```python
from build123d import *

# Parameters (mm, degrees)
F0_W      = 381
F0_H      = 609.6
F1_DEPTH  = 127
F2_T      = -1.5748
F3_W      = 1.5748
F3_H      = 606.4504
F4_DEPTH  = 125.4252
F5_W      = 63.5
F5_H      = 63.5
F6_DEPTH  = 127
F7_W      = 63.5
F7_H      = 63.5
F8_DEPTH  = 128.5748
F9_R      = 22.479
F10_DEPTH = 41.148
F11_R     = 15.875
F12_DEPTH = 42.7228


with BuildPart() as f1:
    # F0 (on Top) → F1 (new body)
    with BuildSketch(Plane.XY):
        with Locations((190.5, 304.8)):
            Rectangle(F0_W, F0_H)
    extrude(amount=F1_DEPTH)

    # F2
    f2_openings = [f1.faces().sort_by_distance(p)[0] for p in [
        (190.5, 304.8, 127),
    ]]
    offset(amount=F2_T, openings=f2_openings)

    # F3 (on face) → F4 (join, through all)
    with BuildSketch(Plane.XY.offset(1.5748)):
        with Locations((129.3622, 304.8)):
            Rectangle(F3_W, F3_H)
        with Locations((256.3622, 304.8)):
            Rectangle(F3_W, F3_H)
    extrude(amount=F4_DEPTH)

    # F5 (on face) → F6 (cut, through all)
    with BuildSketch(Plane.YZ.offset(257.1496)):
        with Locations((33.3248, 33.3248)):
            Rectangle(F5_W, F5_H)
    extrude(amount=-F6_DEPTH, mode=Mode.SUBTRACT)

    # F7 (on face) → F8 (cut, through all)
    with BuildSketch(Plane.YZ.offset(130.1496)):
        with Locations((576.2752, 33.3248)):
            Rectangle(F7_W, F7_H)
    extrude(amount=-F8_DEPTH, mode=Mode.SUBTRACT)

    # F9 (on face) → F10 (join)
    with BuildSketch(Plane(origin=(0, 0, 0), x_dir=(0, -1, 0), z_dir=(-1, 0, 0))):
        with Locations((-22.479, 22.479)):
            Circle(F9_R)
    extrude(amount=F10_DEPTH)

    # F11 (on face) → F12 (cut, through all)
    with BuildSketch(Plane(origin=(-41.148, 0, 0), x_dir=(0, -1, 0), z_dir=(-1, 0, 0))):
        with Locations((-22.479, 22.479)):
            Circle(F11_R)
    extrude(amount=-F12_DEPTH, mode=Mode.SUBTRACT)


solid = f1.part
```
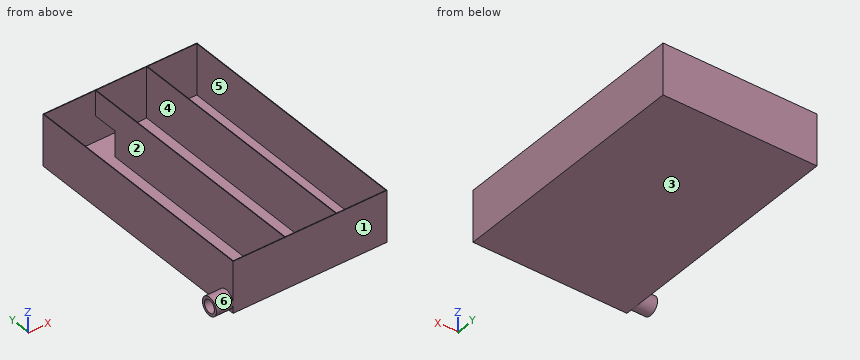
Here's how the part is built. I have some questions about the finished solid (model axes, mm). Face numbers are marked on the shaded views. A direction names the side the tool comes from. Give positions to 0.01 mm unless a question says otherwise; leave off trailing zeros. Write each loop counter-clockwise with the first axis right and the second up, starting at its lowest first coordinate (ties: lowest second). Pieces come first, ordered by that corner, then holes. Notation, with made-up numbers: (88, 40.5) -> (134, 40.5) arc R29 cw to (134, 68.5) -> close; hole circle Ø2 at (-38, 25.25). An arc over 180 degrees is marked (long way). Use one line per item in the form item = value.
1) Suppose I cut it at D-D (y = 370). Please give me the cut outline in (x, z), and give its area (3 significant figures).
Verdict:
outline = (0, 0) -> (381, 0) -> (381, 127) -> (379.43, 127) -> (379.43, 1.57) -> (257.15, 1.57) -> (257.15, 127) -> (255.57, 127) -> (255.57, 1.57) -> (130.15, 1.57) -> (130.15, 127) -> (128.57, 127) -> (128.57, 1.57) -> (1.57, 1.57) -> (1.57, 127) -> (0, 127) -> close
area = 1,390 mm2
2) I'm going to push flat-ended pins straight in: pin 1 (5 mm diameter, centred on y = 281, z = 53.5, fed in from -X); pin 2 (19 mm diameter, centred on y = 22.479, z = 22.479, fed in from -X). Where does each tip first touch, or does it pass through?
Verdict:
pin_1 = 0
pin_2 = 128.57
3) On a 3-axis mill with a long thin cutter (end or side, diameter ignored), from which of +Z, -Z, +X, -X, +Y, -Y can I reach the whole of each face in a straight line? I mean the marked faces 1 and 2. Say none if no direction works.
Verdict:
face_1 = +Z, -Z, +X, -X, -Y
face_2 = +Z
4) If I drill on L1, parallel to X at y = 72, z = 103; L2, parallel to X at y = 582.5, z = 48.5; L3, parallel to X at y = 41, z = 11, over which ranges is the centre line in solid material (lowest first)? Write a range as [from, to].
Verdict:
L1 = [0, 1.57], [128.57, 130.15], [255.57, 257.15], [379.43, 381]
L2 = [0, 1.57], [255.57, 257.15], [379.43, 381]
L3 = [-41.15, 1.57], [128.57, 130.15], [379.43, 381]
5) Suppose I cut it at A-A (y = 566.5). Please give me the cut outline in (x, z), and give its area (3 significant figures).
Verdict:
outline = (0, 0) -> (381, 0) -> (381, 127) -> (379.43, 127) -> (379.43, 1.57) -> (257.15, 1.57) -> (257.15, 127) -> (255.57, 127) -> (255.57, 1.57) -> (1.57, 1.57) -> (1.57, 127) -> (0, 127) -> close; (128.57, 65.07) -> (130.15, 65.07) -> (130.15, 127) -> (128.57, 127) -> close
area = 1,290 mm2
6) Suppose I cut it at C-C (x = 303). Please give me the cut outline in (y, z).
Verdict:
outline = (0, 0) -> (609.6, 0) -> (609.6, 127) -> (608.03, 127) -> (608.03, 1.57) -> (1.57, 1.57) -> (1.57, 127) -> (0, 127) -> close
7) Suppose I cut it at B-B (z = 90.5). Please give me the cut outline in (x, y).
Verdict:
outline = (0, 0) -> (381, 0) -> (381, 609.6) -> (0, 609.6) -> close; hole (1.57, 1.57) -> (128.57, 1.57) -> (128.57, 608.03) -> (1.57, 608.03) -> close; hole (130.15, 1.57) -> (255.57, 1.57) -> (255.57, 608.03) -> (130.15, 608.03) -> close; hole (257.15, 1.57) -> (379.43, 1.57) -> (379.43, 608.03) -> (257.15, 608.03) -> close
8) We'd pull the mould along Y, two halves only. Please class the marked faces 3, 4, 5 and 6: +Y half, -Y half, draft (parallel to the pull), parting line (faces both ways), or undercut.
Verdict:
face_3 = draft
face_4 = undercut
face_5 = undercut
face_6 = parting line
